```python
from build123d import *

# Parameters (mm, degrees)
F2_R     = 10.5
F3_DEPTH = 25
F2_R_2   = 11.5
F4_DEPTH = 9


with BuildPart() as f1:
    # F0 (on Front) → F1 (revolve)
    with BuildSketch(Plane.XZ):
        Polygon((-5.5, 15), (-5.5, 0), (5.5, 0), (5.5, 15), (3.5, 15), (3.5, 13), (-3.5, 13), (-3.5, 15), align=None)
    revolve(axis=Axis((0, 0, 0), (1, 0, 0)))

    # F2 (on face) → F3 (cut)
    with BuildSketch(Plane.YZ.offset(5.5)):
        Circle(F2_R)
    extrude(amount=-F3_DEPTH, mode=Mode.SUBTRACT)

    # F2 (on face) → F4 (cut)
    with BuildSketch(Plane.YZ.offset(5.5)):
        Circle(F2_R_2)
        Circle(F2_R, mode=Mode.SUBTRACT)
    extrude(amount=-F4_DEPTH, mode=Mode.SUBTRACT)


solid = f1.part
```
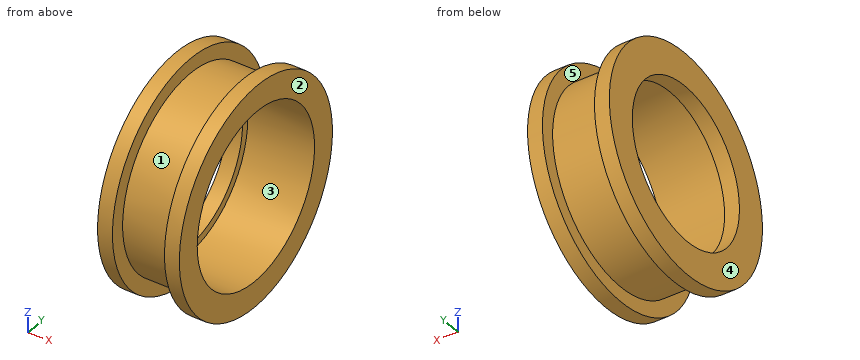
Could you check a few things on this model? Use its own coordinates, in mm. Face numbers are marked on the shaded views. A direction names the side the tool comes from. Round coordinates to 2 decimals unless told otherwise and drop trailing zeros. Write each loop counter-clockwise with the first axis right and the second up, starting at its lowest first coordinate (ties: lowest second). Pieces come first, ordered by that corner, then holes. Notation, with made-up numbers: M -26.5,68 L 16.5,68 A22 cw 16.5,75 Z; hole C -30.75,57.25 d7. An arc over 180 degrees is marked long. Answer in a Markdown table with one row per item. Add a question column.
Q1. If we mould it in two halves opening along Y, with no side actions, what happens to the marked faces 1, 2 and 3? For each: +Y half, -Y half, draft (parallel to the pull), parting line (faces both ways), or undercut.
Q2. Imagine slicing it at A-A (y = 0). Please give me the cut outline in (x, z), then the cut area to 3 significant figures.
Q3. Imagine slicing it at B-B (z = 6.5). Please give me the cut outline in (x, y), then the cut area to 3 significant figures.
Q4. On a 3-axis mill with a long thin cutter (end or side, diameter ignored), from which of +Z, -Z, +X, -X, +Y, -Y can I reach the whole of each face in a straight line? I mean the marked faces 4 and 5. Say none if no direction works.
Q5. Imagine slicing it at D-D (x = 4). Please give me the cut outline in (y, z).
Q6. Imagine slicing it at C-C (x = -2.25). Please give me the cut outline in (y, z).
Q7. If I drill on line 1 (Z direction, x = -4.6, y = 0); line 2 (Z direction, x = -0.5, y = 0); line 3 (X direction, y = 12.25, z = 5.25), over which ranges is the centre line in solid material (lowest first)? Write a range as from..to.
Q8. Will these pins go through, and if not, where does the flat tip stop? pin 1 Ø6 at (x, y) = (-2.5, -9) entering from -Z; pin 2 Ø1 at (x, y) = (2, 4) entering from +Z; pin 3 Ø1.5 at (x, y) = (-4.5, 3.5) entering from +Z.
Values:
| question | item | result |
|---|---|---|
| 1 | face 1 | parting line |
| 1 | face 2 | draft |
| 1 | face 3 | undercut |
| 2 | outline | M -5.5,-15 L -3.5,-15 L -3.5,-13 L 3.5,-13 L 3.5,-15 L 5.5,-15 L 5.5,-11.5 L -3.5,-11.5 L -3.5,-10.5 L -5.5,-10.5 Z; M -5.5,10.5 L -3.5,10.5 L -3.5,11.5 L 5.5,11.5 L 5.5,15 L 3.5,15 L 3.5,13 L -3.5,13 L -3.5,15 L -5.5,15 Z |
| 2 | area | 53.0 mm^2 |
| 3 | outline | M -5.5,-13.52 L -3.5,-13.52 L -3.5,-11.26 L 3.5,-11.26 L 3.5,-13.52 L 5.5,-13.52 L 5.5,-9.49 L -3.5,-9.49 L -3.5,-8.25 L -5.5,-8.25 Z; M -5.5,8.25 L -3.5,8.25 L -3.5,9.49 L 5.5,9.49 L 5.5,13.52 L 3.5,13.52 L 3.5,11.26 L -3.5,11.26 L -3.5,13.52 L -5.5,13.52 Z |
| 3 | area | 62.0 mm^2 |
| 4 | face 4 | +Z, -Z, -X, +Y, -Y |
| 4 | face 5 | none |
| 5 | outline | C 0,0 d30; hole C 0,0 d23 |
| 6 | outline | C 0,0 d26; hole C 0,0 d23 |
| 7 | line 1 | -15..-10.5, 10.5..15 |
| 7 | line 2 | -13..-11.5, 11.5..13 |
| 7 | line 3 | -5.5..-3.5, 3.5..5.5 |
| 8 | pin 1 | z = -13.67 |
| 8 | pin 2 | z = 12.52 |
| 8 | pin 3 | z = 14.75 |
